Model file for the job. Use its own axes, mm. Coordinates: 2 decimals unless noted, no trailing zeros. Order: outer loops, then holes, each group sorted by start corner. A loop starts at its lowest first (then second) coordinate and runs counter-clockwise, first axis right, second up.
from build123d import *

# Parameters (mm, degrees)
BOSS_EXTRUDE2_DEPTH   = 4.7625
F_4_CLEARANCE_HOLE1_D = 3.2639
SKETCH5_R             = 3.1623
CUT_EXTRUDE1_DEPTH    = 5.7625


with BuildPart() as part:
    # Sketch1 → Boss-Extrude2 (new body)
    with BuildSketch(Plane(origin=(0, 0, 0), x_dir=(1, 0, 0), z_dir=(0, 1, 0))):
        with BuildLine():
            Line((-63.5, 6.35), (0, 6.35))
            ThreePointArc((0, 6.35), (6.35, 0), (0, -6.35))
            Line((0, -6.35), (-63.5, -6.35))
            ThreePointArc((-63.5, -6.35), (-69.85, 0), (-63.5, 6.35))
        make_face()
    extrude(amount=BOSS_EXTRUDE2_DEPTH)

    # #4 Clearance Hole1 (through all)
    with Locations(Plane(origin=(0, 4.7625, 0), x_dir=(1, 0, 0), z_dir=(0, 1, 0))):
        with Locations((0, 0)):
            Hole(F_4_CLEARANCE_HOLE1_D / 2)

    # Sketch5 → Cut-Extrude1 (cut, through all)
    with BuildSketch(Plane(origin=(0, 4.7625, 0), x_dir=(1, 0, 0), z_dir=(0, 1, 0))):
        with Locations((-63.5, 0)):
            Circle(SKETCH5_R)
    extrude(amount=-CUT_EXTRUDE1_DEPTH, mode=Mode.SUBTRACT)


solid = part.part
Q1. Mould opens along X. For faces 1 (the face through (6.35, 2.35, -0.14)), 2 (the face through (-31, 4.762, 0)), 3 (the face through (-66.66, 2.41, -0.14)) say: pulls with the +X half, pulls with the -X half, needs draft (parallel to the pull), parting line crosses it, or undercut.
Established:
face 1: pulls with the +X half
face 2: needs draft
face 3: undercut
Q2. Cut at C-C, the plane z = 5.25. List the corners of the cut face in (x, y).
Established:
outline: (-67.07, 0) - (3.57, 0) - (3.57, 4.76) - (-67.07, 4.76) - close
Q3. Drop flat-ended pins along their axis: P1, Ø1, axis at y = 3.5, z = 3.5, coming from the +X side; P2, Ø2, axis at x = 0, z = 0, coming from the +Y side. Give the stop position or say it passes through.
Established:
P1: stops at x = 5.6
P2: passes through
Q4. Cut at B-B, the plane y = 1.4. List the corners of the cut face in (x, z).
Established:
outline: (-63.5, -6.35) - (0, -6.35) arc R6.35 ccw to (0, 6.35) - (-63.5, 6.35) arc R6.35 ccw to start; hole circle Ø6.32 at (-63.5, 0); hole circle Ø3.26 at (0, 0)
Q5. Cut at A-A, the plane z = 0. List the corners of the cut face in (x, y), plus the area to 3 significant figures.
Established:
outline: (-69.85, 0) - (-66.66, 0) - (-66.66, 4.76) - (-69.85, 4.76) - close; (-60.34, 0) - (-1.63, 0) - (-1.63, 4.76) - (-60.34, 4.76) - close; (1.63, 0) - (6.35, 0) - (6.35, 4.76) - (1.63, 4.76) - close
area: 317 mm2
Q6. Cut at D-D, the plane z = -4.25. List the corners of the cut face in (x, y), plus the area to 3 significant figures.
Established:
outline: (-68.22, 0) - (4.72, 0) - (4.72, 4.76) - (-68.22, 4.76) - close
area: 347 mm2
Q7. Probe line 1 (Z direction, x = -63.5, y = 1.75); line 2 (X direction, y = 1.8, z = -0.25); line 3 (X direction, y = 2.25, z = -1.75). List the from-to ranges inside material, lowest first.
Established:
line 1: z = -6.35 to -3.16, 3.16 to 6.35
line 2: x = -69.85 to -66.65, -60.35 to -1.61, 1.61 to 6.35
line 3: x = -69.6 to -66.13, -60.87 to 6.1
